Autodesk Inventor part; units mm, degrees
ref_plane "YZ Plane" through (0, 0, 0) normal (1, 0, 0) x (0, 1, 0)
ref_plane "XZ Plane" through (0, 0, 0) normal (0, 1, 0) x (-1, 0, 0)
ref_plane "XY Plane" through (0, 0, 0) normal (0, 0, 1) x (1, 0, 0)
sketch "Sketch1" plane through (0, 0, 0) normal (0, 0, 1) x (1, 0, 0)
  circle A0 centre (14.22, 3.81) radius 1.5
  circle A1 centre (14.22, -4.69) radius 1.5
  line L0 (8.6298, -8.5) -> (19.8102, -8.5)
  line L1 (19.8102, -8.5) -> (19.8102, 0)
  line L2 (19.8102, 0) -> (8.6298, 0)
  line L3 (8.6298, 0) -> (8.6298, -8.5)
  line L4 (8.6298, 0) -> (19.8102, 0)
  line L5 (19.8102, 0) -> (19.8102, 7.62)
  line L6 (19.8102, 7.62) -> (8.6298, 7.62)
  line L7 (8.6298, 7.62) -> (8.6298, 0)
  point P0 (0, 0)
  dimension "d0" = 3.81
extrude "Extrusion1" add sketch "Sketch1" along normal blind 4.5 contours L7 L6 L5 L2
fillet "Fillet1" radius 1 4 edges at (8.6298, 7.62, 2.25) (8.6298, 0, 2.25) (19.8102, 7.62, 2.25) (19.8102, 0, 2.25)
properties part number "ConnectingBlockTail"
Geometry: final body of the model. Coordinates: model frame, mm. Give positions to 0.01 mm unless a question says otherwise; leave off trailing zeros. Loops run counter-clockwise (first coordinate to the right, second up) from the corner with the lowest first, then second, coordinate; pieces in that order, holes last. Notation, with made-up numbers: M 2,55.25 L 58,55.25 A15 cw 58,60.25 Z; hole C -27.5,10 d10. An arc over 180 degrees is marked long. Put each result on its own line as item: value.
1) Cut plane A-A, the plane x = 14.22. Return the cut outline in (y, z).
Computed values:
outline: M 0,0 L 2.31,0 L 2.31,4.5 L 0,4.5 Z; M 5.31,0 L 7.62,0 L 7.62,4.5 L 5.31,4.5 Z
2) Mould query, pull axis X, two halves, no side actions, for faces 1 (the cylindrical face through (12.72, 3.74, 2.22)), 2 (the flat face through (14, 7.62, 2)), 3 (the cylindrical face through (8.915, 0.301, 2.282)). Classes: released by +X, released by -X, zero draft, split by the parting line, or undercut.
Computed values:
face 1: undercut
face 2: zero draft
face 3: released by -X
3) Material intervals for L1, parallel to Y at x = 14.22, z = 1.25; L2, parallel to Y at x = 15.25, z = 2.3; L3, parallel to X at y = 2.5, z = 2.1, sorted ascending. Write a range as from..to.
Computed values:
L1: y = 0..2.31, 5.31..7.62
L2: y = 0..2.72, 4.9..7.62
L3: x = 8.63..13.49, 14.95..19.81
4) Cut plane B-B, the plane y = 3.81. Return the cut outline in (x, z), plus the area to 3 significant figures.
Computed values:
outline: M 8.63,0 L 12.72,0 L 12.72,4.5 L 8.63,4.5 Z; M 15.72,0 L 19.81,0 L 19.81,4.5 L 15.72,4.5 Z
area: 36.8 mm^2
5) Cut plane C-C, the plane z = 2.4. Return the cut outline in (x, y), plus the area to 3 significant figures.
Computed values:
outline: M 8.63,1 A1 ccw 9.63,0 L 18.81,0 A1 ccw 19.81,1 L 19.81,6.62 A1 ccw 18.81,7.62 L 9.63,7.62 A1 ccw 8.63,6.62 Z; hole C 14.22,3.81 d3
area: 77.3 mm^2
